Geometry: final body of the model. Coordinates: model frame, mm. A direction names the side the tool comes from. Give positions to 0.01 mm unless a question says otherwise; leave off trailing zeros. Order: outer loops, then holes, each group sorted by start corner. A loop starts at its lowest first (then second) coordinate and runs counter-clockwise, first axis right, second up. Notation, with made-up numbers: (23, 64.25) -> (63, 64.25) arc R28 ccw to (63, 101.25) -> close; hole circle Ø4 at (70.5, 59). An arc over 180 degrees is marked (long way). Write item = value, one per line.
```python
from build123d import *

# Parameters (mm, degrees)
SKETCH_1_R               = 9.17
EXTRUDE_1_DEPTH          = 11
CUT_EXTRUDE_1_DEPTH      = 11
PATTERN_CIRCULAR_1_COUNT = 20
SKETCH_4_R               = 11
EXTRUDE_3_DEPTH          = 8
EXTRUDE_START            = 1
SKETCH_3_R               = 11
EXTRUDE_4_DEPTH          = 1
SKETCH_5_R               = 2.5
CUT_EXTRUDE_2_DEPTH      = 22
SKETCH_6_R               = 1.5
CUT_EXTRUDE_3_DEPTH      = 30


with BuildPart() as part:
    # 草图1 → 凸台-拉伸1 (new body)
    with BuildSketch(Plane(origin=(0, 0, 0), x_dir=(1, 0, 0), z_dir=(0, 1, 0))):
        with Locations(Location((0, 0, 0), (0, 0, 270))):
            Circle(SKETCH_1_R)
    extrude(amount=-EXTRUDE_1_DEPTH)

    # 草图2 → 切除-拉伸1 (cut)
    with BuildSketch(Plane(origin=(0, 0, 0), x_dir=(1, 0, 0), z_dir=(0, 1, 0))):
        with BuildLine():
            Line((-1.338469592, 9.071791397), (-1.301979145, 9.548134799))
            Line((-1.301979145, 9.548134799), (1.164461041, 9.508969944))
            Line((1.164461041, 9.508969944), (1.338469592, 9.071791397))
            ThreePointArc((1.338469592, 9.071791397), (1.164461041, 9.03324808), (1.06034373, 8.888596261))
            ThreePointArc((1.06034373, 8.888596261), (0, 8.072950826), (-1.06034373, 8.888596261))
            ThreePointArc((-1.06034373, 8.888596261), (-1.164461041, 9.03324808), (-1.338469592, 9.071791397))
        make_face()
    cut_extrude_1 = extrude(amount=-CUT_EXTRUDE_1_DEPTH, mode=Mode.SUBTRACT)

    # 阵列(圆周)1: 切除-拉伸1 ×20 about axis
    pattern_circular_1_axis = Axis((0, 0, 0), (0, 1, 0))
    for i in range(1, PATTERN_CIRCULAR_1_COUNT):
        add(cut_extrude_1.rotate(pattern_circular_1_axis, i * 360 / PATTERN_CIRCULAR_1_COUNT), mode=Mode.SUBTRACT)

    # 草图4 → 凸台-拉伸3 (add)
    with BuildSketch(Plane(origin=(0, 0, 0), x_dir=(1, 0, 0), z_dir=(0, 1, 0))):
        with Locations(Location((0, 0, 0), (0, 0, 270))):
            Circle(SKETCH_4_R)
    extrude(amount=EXTRUDE_3_DEPTH)

    # 草图3 → 凸台-拉伸4 (add)
    with BuildSketch(Plane.XZ.offset(11).offset(EXTRUDE_START)):
        with Locations(Location((0, 0, 0), (0, 0, 90))):
            Circle(SKETCH_3_R)
    extrude(amount=-EXTRUDE_4_DEPTH)

    # 草图5 → 切除-拉伸2 (cut)
    with BuildSketch(Plane(origin=(0, 8, 0), x_dir=(1, 0, 0), z_dir=(0, 1, 0))):
        with Locations(Location((0, 0, 0), (0, 0, 270))):
            Circle(SKETCH_5_R)
    extrude(amount=-CUT_EXTRUDE_2_DEPTH, mode=Mode.SUBTRACT)

    # 草图6 → 切除-拉伸3 (cut)
    with BuildSketch(Plane.XY):
        with Locations((0, 4)):
            Circle(SKETCH_6_R)
    extrude(amount=-CUT_EXTRUDE_3_DEPTH, mode=Mode.SUBTRACT)


solid = part.part
```
1) First-contact query: P1, Ø5, axis at x = -1, y = -7.5, coming from the -Z side; P2, Ø11, axis at x = 0.5, z = 2, coming from the +Y side; P3, Ø5, axis at y = -8, z = 0, coming from the -X side; P4, Ø8, axis at y = -2.5, z = -4, coming from the -X side. Flat tips, straight axial feed; report the tip coordinate or a pass-through.
Check sheet entries:
P1 = -9.07
P2 = 8
P3 = -9.07
P4 = -10.96
2) Line query: line 1 (Y direction, x = 8.75, z = 5.5); line 2 (X direction, y = -2.5, z = -3.75); line 3 (Z direction, x = -0.25, y = -5.25). Output: solid intervals per line, ascending. Write a range as from..to.
Check sheet entries:
line_1 = -12..-11, 0..8
line_2 = -8.12..8.12
line_3 = -8.1..-2.49, 2.49..8.1
3) Mould query, pull axis Z, two halves, no side actions, for faces 1 (the face through (0, 8, -3)), 2 (the face through (-8.073, -5.423, -0.02)), 3 (the face through (10.74, -11.51, -2.38)). Classes: +Z half, -Z half, draft (parallel to the pull), parting line (faces both ways), or undercut.
Check sheet entries:
face_1 = draft
face_2 = undercut
face_3 = parting line
4) Section query B-B (x = 0). Output: boundary loops of the cut face in (y, z).
Check sheet entries:
outline = (-12, -11) -> (-11, -11) -> (-11, -8.07) -> (0, -8.07) -> (0, -11) -> (2.5, -11) -> (2.5, -2.5) -> (-12, -2.5) -> close; (-12, 2.5) -> (8, 2.5) -> (8, 11) -> (0, 11) -> (0, 8.07) -> (-11, 8.07) -> (-11, 11) -> (-12, 11) -> close; (5.5, -11) -> (8, -11) -> (8, -2.5) -> (5.5, -2.5) -> close
5) Section query D-D (y = 6.5). Output: boundary loops of the cut face in (x, z), plus the area to 3 significant figures.
Check sheet entries:
outline = circle Ø22 at (0, 0); hole circle Ø5 at (0, 0)
area = 360 mm²
6) Section query C-C (z = -7). Output: boundary loops of the cut face in (x, y).
Check sheet entries:
outline = (-8.49, -12) -> (8.49, -12) -> (8.49, -11) -> (4.38, -11) -> (4.38, 0) -> (8.49, 0) -> (8.49, 8) -> (-8.49, 8) -> (-8.49, 0) -> (-4.38, 0) -> (-4.38, -11) -> (-8.49, -11) -> close; hole circle Ø3 at (0, 4)
7) Section query A-A (z = 0). Output: boundary loops of the cut face in (x, y).
Check sheet entries:
outline = (-11, -12) -> (-2.5, -12) -> (-2.5, 8) -> (-11, 8) -> (-11, 0) -> (-8.07, 0) -> (-8.07, -11) -> (-11, -11) -> close; (2.5, -12) -> (11, -12) -> (11, -11) -> (8.07, -11) -> (8.07, 0) -> (11, 0) -> (11, 8) -> (2.5, 8) -> close
8) Reachability of faces 4 (the face through (0.751, -1.86, 2.385)), 5 (the face through (1.43, 4.45, -6.44)), 6 (the face through (6.54, -5.42, -4.73)), 7 (the face through (8.073, -5.423, 0.02)) from +Z, -Z, +X, -X, +Y, -Y: full face, straight path, thin tool, end or side. Return the list, or none.
Check sheet entries:
face_4 = +Y, -Y
face_5 = -Z
face_6 = none
face_7 = +X
